Can you work these out from the model? Positions are in its coordinate system, mm. Face numbers are marked on the shaded views. A direction names the side the tool comes from. Coordinates: 2 decimals unless noted, no trailing zeros. Order: outer loops, then holes, each group sorted by start corner. A loop starts at its lowest first (then second) coordinate and runs counter-clockwise, first axis right, second up. Notation, with made-up numbers: (37, -4.75) -> (79, -4.75) arc R24 ccw to (79, 7.25) -> close; hole circle Ø5 at (-12, 52.25). An arc over 180 degrees is marked (long way). Write item = value, one per line.
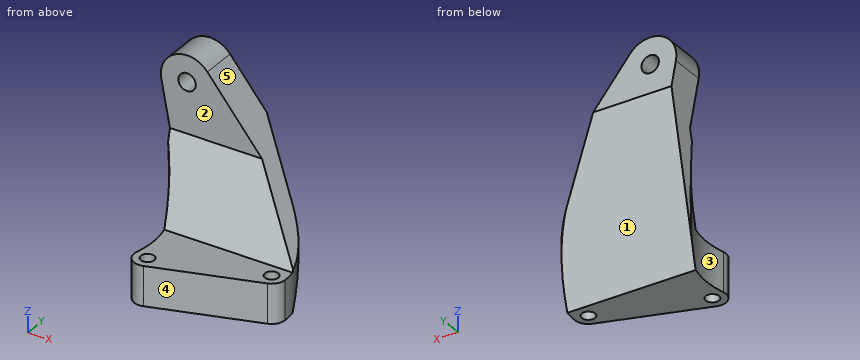
```python
from build123d import *

# Parameters (mm, degrees)
SKETCH1_R            = 1.55
BOSS_EXTRUDE1_DEPTH  = 9
BOSS_EXTRUDE12_DEPTH = 17.39274351
SKETCH7_3_OUTSIDE_W  = 51.494
SKETCH7_3_OUTSIDE_H  = 57.894
SKETCH7_3_OUTSIDE_R  = 2
CUT_EXTRUDE3_DEPTH   = 17.39274351
CUT_EXTRUDE2_DEPTH   = 50
CUT_EXTRUDE5_DEPTH   = 58.797577804
CUT_EXTRUDE7_DEPTH   = 58.797577804
SKETCH15_W           = 41.045636652
SKETCH15_H           = 32.401588668
CUT_EXTRUDE8_DEPTH   = 58.797577804


with BuildPart() as part:
    # Sketch1 → Boss-Extrude1 (new body)
    with BuildSketch(Plane.XY):
        with BuildLine():
            Line((26.6, 7.50725649), (26.6, 10.60725649))
            Line((26.6, 10.60725649), (-3.1, 10.60725649))
            Line((-3.1, 10.60725649), (-3.1, 0))
            ThreePointArc((-3.1, 0), (-1.828333755, -2.503436774), (0.943352052, -2.952979327))
            Line((0.943352052, -2.952979327), (24.443352052, 4.554277162))
            ThreePointArc((24.443352052, 4.554277162), (26.003436774, 5.678922735), (26.6, 7.50725649))
        make_face()
        Circle(SKETCH1_R, mode=Mode.SUBTRACT)
        with Locations((23.5, 7.50725649)):
            Circle(SKETCH1_R, mode=Mode.SUBTRACT)
    extrude(amount=-BOSS_EXTRUDE1_DEPTH)

    # Sketch7 → Boss-Extrude12 (add)
    with BuildSketch(Plane(origin=(0, 28, 0), x_dir=(1, 0, 0), z_dir=(0, 1, 0))):
        with BuildLine():
            Line((-3.1, 0), (-9.895228332, 35.883629581))
            ThreePointArc((-9.895228332, 35.883629581), (-6.533149103, 42.439039954), (0.648143683, 40.794042739))
            Line((0.648143683, 40.794042739), (26.6, 9))
            Line((26.6, 9), (26.6, 0))
            Line((26.6, 0), (-3.1, 0))
        make_face()
    extrude(amount=-BOSS_EXTRUDE12_DEPTH)

    # Sketch7<3> outside → Cut-Extrude3 (cut)
    # profile 1 of 2: a face of its own
    with BuildSketch(Plane(origin=(0, 28, 0), x_dir=(1, 0, 0), z_dir=(0, 1, 0))):
        with Locations((8.3, 21.5)):
            Rectangle(SKETCH7_3_OUTSIDE_W, SKETCH7_3_OUTSIDE_H)
        with BuildLine():
            Line((-3.1, 0), (-9.895228332, 35.883629581))
            ThreePointArc((-9.895228332, 35.883629581), (-6.533149103, 42.439039954), (0.648143683, 40.794042739))
            Line((0.648143683, 40.794042739), (26.6, 9))
            Line((26.6, 9), (26.6, 0))
            Line((26.6, 0), (-3.1, 0))
        make_face(mode=Mode.SUBTRACT)
    # profile 2 of 2: a face of its own
    with BuildSketch(Plane(origin=(0, 28, 0), x_dir=(1, 0, 0), z_dir=(0, 1, 0))):
        with Locations(Location((-4, 37, 0), (0, 0, 270))):
            Circle(SKETCH7_3_OUTSIDE_R)
    extrude(amount=-CUT_EXTRUDE3_DEPTH, mode=Mode.SUBTRACT)

    # Sketch8 → Cut-Extrude2 (cut, symmetric)
    with BuildSketch(Plane(origin=(0, 0, 0), x_dir=(0, 0, -1), z_dir=(1, 0, 0))):
        Polygon((0, 10.60725649), (30.5, 28), (0, 28), align=None)
        Polygon((43, 20), (25.471160912, 20), (9, 10.60725649), (43, 10.60725649), align=None)
    extrude(amount=CUT_EXTRUDE2_DEPTH, both=True, mode=Mode.SUBTRACT)

    # Sketch12 → Cut-Extrude5 (cut, through all)
    with BuildSketch(Plane.XY):
        with BuildLine():
            Line((-3.1, 0), (-7.493582912, 18.705566962))
            ThreePointArc((-7.493582912, 18.705566962), (-3.016370904, 10.284014045), (-3.008825552, 0.746303421))
            ThreePointArc((-3.008825552, 0.746303421), (-3.077121968, 0.375926049), (-3.1, 0))
        make_face()
    extrude(amount=-CUT_EXTRUDE5_DEPTH, mode=Mode.SUBTRACT)

    # Sketch14 → Cut-Extrude7 (cut, through all)
    with BuildSketch(Plane.XY):
        with BuildLine():
            Line((19.851500316, 20.45422786), (26.6, 15.73954146))
            Line((26.6, 15.73954146), (26.6, 7.50725649))
            ThreePointArc((26.6, 7.50725649), (24.811622249, 14.807364633), (19.851500316, 20.45422786))
        make_face()
    extrude(amount=-CUT_EXTRUDE7_DEPTH, mode=Mode.SUBTRACT)

    # Mirror9: part across plane


with BuildPart() as part_1:
    add(part.part)
    add(part.part.mirror(Plane.XY))

    # Sketch15 → Cut-Extrude8 (cut, through all)
    with BuildSketch(Plane.XY):
        with Locations((9.251388929, 12.77619049)):
            Rectangle(SKETCH15_W, SKETCH15_H)
    extrude(amount=-CUT_EXTRUDE8_DEPTH, mode=Mode.SUBTRACT)


solid = part_1.part
```
Item 1: I'm going to push flat-ended pins straight in: P1, Ø9, axis at x = -0.5, z = 33.5, coming from the -Y side; P2, Ø7, axis at x = 13.5, y = 6, coming from the +Z side; P3, Ø1, axis at x = 10, z = 23.5, coming from the -Y side; P4, Ø3, axis at x = 23.5, y = 7.51, coming from the +Z side. Where does each tip first touch, or does it pass through?
A:
P1 = 20
P2 = 9
P3 = 18.59
P4 = through
Item 2: I want a section at C-C, the plane z = 37. Please give me the cut outline in (x, y).
A:
outline = (-10, 20) -> (-6, 20) -> (-6, 28) -> (-10, 28) -> close; (-2, 20) -> (3.75, 20) -> (3.75, 28) -> (-2, 28) -> close
Item 3: I want a section at B-B, the plane y = 8.5. Please give me the cut outline in (x, z).
A:
outline = (-2.66, 0) -> (22.31, 0) -> (22.31, 9) -> (-2.66, 9) -> close; (24.69, 0) -> (26.57, 0) -> (26.57, 9) -> (24.69, 9) -> close
Item 4: I want a section at A-A, the plane x = -5. Please give me the cut outline in (y, z), plus the area to 4 significant figures.
A:
outline = (15.24, 10.03) -> (16.33, 10.03) -> (28, 30.5) -> (28, 35.27) -> (20, 35.27) -> (20, 25.47) -> (15.24, 17.13) -> close; (20, 38.73) -> (28, 38.73) -> (28, 42.92) -> (20, 42.92) -> close
area = 169.5 mm2
Item 5: If we mould it in two halves opening along Y, with no side actions, what happens to the marked faces 3, 4 and 5? For each: pulls with the +Y half, pulls with the -Y half, needs draft (parallel to the pull), parting line crosses it, or undercut.
A:
face_3 = undercut
face_4 = pulls with the -Y half
face_5 = needs draft
Item 6: I want a section at D-D, the plane y = 25. Please give me the cut outline in (x, z), plus the area to 3 significant figures.
A:
outline = (-9.9, 35.88) -> (-7.88, 25.24) -> (13.34, 25.24) -> (0.65, 40.79) arc R6 ccw to start; hole circle Ø4 at (-4, 37)
area = 253 mm2
Item 7: If I drill on probe 1 along Z at (x, y) = (0.5, 5.5); probe 2 along Y at (x, z) = (-5.5, 34.5); probe 3 along Y at (x, z) = (7, 25.5), over which ranges is the centre line in solid material (lowest first)?
A:
probe_1 = 0 to 9
probe_2 = 20 to 28
probe_3 = 20 to 25.15
Item 8: For the marked faces 1 and 2, which set-ups out of +Z, -Z, +X, -X, +Y, -Y let a thin tool reach every point of the face, with its end or its side?
A:
face_1 = -Z, +X, -X, +Y
face_2 = +Z, +X, -X, -Y
